Check sheet for the modelled part. Datum: model origin and axes. Units: mm. A direction names the side the tool comes from. Round coordinates to 2 decimals unless told otherwise and drop trailing zeros. Order: outer loops, then holes, each group sorted by start corner. A loop starts at its lowest first (then second) coordinate and runs counter-clockwise, first axis right, second up. Notation, with made-up numbers: (-14.5, -1) -> (-9.5, -1) arc R22 ccw to (-9.5, 35) -> close; hole circle Ø1 at (53.25, -24). An arc over 180 degrees is marked (long way). Answer in a Markdown table with one row per item.
from build123d import *

# Parameters (mm, degrees)
F1_DEPTH = 9.525
F2_R     = 2.54
F3_DEPTH = 19.355562
F4_R     = 2.54
F5_DEPTH = 19.051


with BuildPart() as f1:
    # F0 (on Front) → F1 (new body, symmetric)
    with BuildSketch(Plane.XZ):
        Polygon((-9.525, -9.677281), (9.525, -9.677281), (9.525, 9.677281), (5.08, 6.502281), (6.35, 6.502281), (6.35, -6.502281), (-6.35, -6.502281), (-6.35, 6.502281), (-5.08, 6.502281), (-9.525, 9.677281), align=None)
    extrude(amount=F1_DEPTH, both=True)

    # F2 (on face) → F3 (cut, through all)
    with BuildSketch(Plane(origin=(0, 0, -9.677281), x_dir=(1, 0, 0), z_dir=(0, 0, -1))):
        Circle(F2_R)
    extrude(amount=-F3_DEPTH, mode=Mode.SUBTRACT)

    # F4 (on face) → F5 (cut, through all)
    with BuildSketch(Plane.YZ.offset(9.525)):
        Circle(F4_R)
    extrude(amount=-F5_DEPTH, mode=Mode.SUBTRACT)


solid = f1.part
Item 1: Mould release check, pull along Y, two halves, no side actions. Record for faces 1 (the flat face through (-6.5, 9.525, -2)), 2 (the cylindrical face through (-0.33, -2.52, -8.11)), 3 (the flat face through (2, -2, -6.502)): pulls with the +Y half, pulls with the -Y half, needs draft (parallel to the pull), parting line crosses it, or undercut.
Result sheet:
| item | result |
|---|---|
| face 1 | pulls with the +Y half |
| face 2 | undercut |
| face 3 | needs draft |
Item 2: Scan lines: line 1 (X direction, y = 0, z = -8.7) (3 decimals); line 2 (X direction, y = 1.75, z = 3) (3 decimals). Record each from-to range of solid material in increasing order. Write a range as [from, to].
Result sheet:
| item | result |
|---|---|
| line 1 | x = [-9.525, -2.54], [2.54, 9.525] |
| line 2 | x = [-9.525, -6.35], [6.35, 9.525] |
Item 3: Cross-section at B-B (z = 0). Record the boundary of the cut face in (x, y) (3 decimals), and give its area (3 significant figures).
Result sheet:
| item | result |
|---|---|
| outline | (-9.525, -9.525) -> (-6.35, -9.525) -> (-6.35, -2.54) -> (-9.525, -2.54) -> close; (-9.525, 2.54) -> (-6.35, 2.54) -> (-6.35, 9.525) -> (-9.525, 9.525) -> close; (6.35, -9.525) -> (9.525, -9.525) -> (9.525, -2.54) -> (6.35, -2.54) -> close; (6.35, 2.54) -> (9.525, 2.54) -> (9.525, 9.525) -> (6.35, 9.525) -> close |
| area | 88.7 mm^2 |
Item 4: Cross-section at A-A (x = 0). Record the boundary of the cut face in (y, z) (3 decimals), and give its area (3 significant figures).
Result sheet:
| item | result |
|---|---|
| outline | (-9.525, -9.677) -> (-2.54, -9.677) -> (-2.54, -6.502) -> (-9.525, -6.502) -> close; (2.54, -9.677) -> (9.525, -9.677) -> (9.525, -6.502) -> (2.54, -6.502) -> close |
| area | 44.4 mm^2 |
Item 5: Set-up check for faces 4 (the flat face through (6, 0, 6.502)), 5 (the flat face through (-9.525, -2, 2)), 6 (the flat face through (-7.271, -0.133, 8.068)): record each of +Z, -Z, +X, -X, +Y, -Y from which the full face is reachable in a straight line by a thin tool's end or side.
Result sheet:
| item | result |
|---|---|
| face 4 | +Y, -Y |
| face 5 | +Z, -Z, -X, +Y, -Y |
| face 6 | +Z, +Y, -Y |
Item 6: Cross-section at C-C (y = 0). Record the boundary of the cut face in (x, z) (3 decimals), and give its area (3 significant figures).
Result sheet:
| item | result |
|---|---|
| outline | (-9.525, -9.677) -> (-2.54, -9.677) -> (-2.54, -6.502) -> (-6.35, -6.502) -> (-6.35, -2.54) -> (-9.525, -2.54) -> close; (-9.525, 2.54) -> (-6.35, 2.54) -> (-6.35, 6.502) -> (-5.08, 6.502) -> (-9.525, 9.677) -> close; (2.54, -9.677) -> (9.525, -9.677) -> (9.525, -2.54) -> (6.35, -2.54) -> (6.35, -6.502) -> (2.54, -6.502) -> close; (5.08, 6.502) -> (6.35, 6.502) -> (6.35, 2.54) -> (9.525, 2.54) -> (9.525, 9.677) -> close |
| area | 109 mm^2 |
Item 7: Depth check by flat-ended pin: P1, Ø8, axis at x = 5.5, y = -7, coming from the +Z side; P2, Ø5, axis at x = 5.5, y = 7, coming from the +Z side. Enter the tip coordinate at first touch or a pass-through.
Result sheet:
| item | result |
|---|---|
| P1 | stops at z = 9.66 |
| P2 | stops at z = 8.59 |
Item 8: Cross-section at D-D (y = 7.25). Record the boundary of the cut face in (x, z) (3 decimals).
Result sheet:
| item | result |
|---|---|
| outline | (-9.525, -9.677) -> (9.525, -9.677) -> (9.525, 9.677) -> (5.08, 6.502) -> (6.35, 6.502) -> (6.35, -6.502) -> (-6.35, -6.502) -> (-6.35, 6.502) -> (-5.08, 6.502) -> (-9.525, 9.677) -> close |
